```python
from build123d import *

# Parameters (mm, degrees)
F1_DEPTH = 10


with BuildPart() as f1:
    # F0 (on Top) → F1 (new body, symmetric)
    with BuildSketch(Plane.XY):
        Polygon((-12.415687, 121.606898), (5.389277, 130.716414), (-27.5, 195), (-46.656741, 188.532595), align=None)
        Polygon((7.5, 82.680783), (7.5, 126.590909), (5.389277, 130.716414), (-12.415687, 121.606898), align=None)
        Polygon((7.5, 0), (27.5, 0), (27.5, 87.5), (7.5, 126.590909), (7.5, 82.680783), align=None)
        Polygon((27.5, -87.5), (27.5, 0), (7.5, 0), (7.5, -82.680783), (-17.804963, -132.140484), (0, -141.25), align=None)
        Polygon((-27.5, -195), (0, -141.25), (-17.804963, -132.140484), (-45.884107, -187.022447), align=None)
    extrude(amount=F1_DEPTH, both=True)


solid = f1.part
```
Input: part model. Units: mm. Frame: model coordinates. Coordinates: 2 decimals unless noted, no trailing zeros. Write each loop counter-clockwise with the first axis right and the second up, starting at its lowest first coordinate (ties: lowest second). Pieces come first, ordered by that corner, then holes.
1) Section A-A on z = -6. Output: boundary loops of the cut face in (x, y), and give its area (3 significant figures).
2) Section B-B on x = -32. Output: boundary loops of the cut face in (y, z), and give its area (3 significant figures).
3) Mould query, pull axis Y, two halves, no side actions, for faces 1 (the flat face through (-36.821, -190.955, 0.14)), 2 (the flat face through (-36.944, 191.812, 0.14)), 3 (the flat face through (7.5, 1, 0)), 4 (the flat face through (12, 1, 10)). Classes: pulls with the +Y half, pulls with the -Y half, needs draft (parallel to the pull), parting line crosses it, or undercut.
4) Pin query (flat end, axial travel): pin 1 Ø1 at (x, z) = (-12, 7) entering from -Y; pin 2 Ø3 at (y, z) = (94.5, 0.5) entering from +X; pin 3 Ø10 at (y, z) = (-24.5, -3.5) entering from -X. Return the tip coordinate at first contact, or that it passes through.
5) Material intervals for line 1 along X through (y, z) = (-5.5, 2); line 2 along Y through (x, z) = (-23.5, 0.25); line 3 along Y through (x, z) = (-13.5, 4.5), sorted ascending.
6) Section C-C on y = 32. Output: boundary loops of the cut face in (x, z).
7) Section D-D on x = 15. Output: boundary loops of the cut face in (y, z), and give its area (3 significant figures).
Check result:
1. outline: (-46.66, 188.53) - (7.5, 82.68) - (7.5, -82.68) - (-45.88, -187.02) - (-27.5, -195) - (27.5, -87.5) - (27.5, 87.5) - (-27.5, 195) - close
1. area: 8,180 mm2
2. outline: (-193.05, -10) - (-159.89, -10) - (-159.89, 10) - (-193.05, 10) - close; (159.89, -10) - (193.48, -10) - (193.48, 10) - (159.89, 10) - close
2. area: 1,340 mm2
3. face 1: pulls with the -Y half
3. face 2: pulls with the +Y half
3. face 3: undercut
3. face 4: needs draft
4. pin 1: stops at y = -165.68
4. pin 2: stops at x = 24.69
4. pin 3: stops at x = 7.5
5. line 1: x = 7.5 to 27.5
5. line 2: y = -187.18 to -143.27, 143.27 to 187.18
5. line 3: y = -167.64 to -123.73, 123.73 to 167.64
6. outline: (7.5, -10) - (27.5, -10) - (27.5, 10) - (7.5, 10) - close
7. outline: (-111.93, -10) - (111.93, -10) - (111.93, 10) - (-111.93, 10) - close
7. area: 4,480 mm2
